Read the model definition and answer for the solid it produces. Units are mm, in the model's axes. A direction names the side the tool comes from. Coordinates: 2 decimals unless noted, no trailing zeros. Order: outer loops, then holes, each group sorted by start corner. A loop starts at its lowest first (then second) coordinate and runs counter-clockwise, first axis right, second up. Notation, with made-up numbers: (38.25, -22) -> (56.25, -22) arc R22 cw to (56.25, -5) -> close; hole circle Ø1 at (21.5, 23). An arc over 180 degrees is marked (long way). Answer in a Markdown table with one row per item.
from build123d import *
from build123d.topology import SkipClean

# Parameters (mm, degrees)
SKETCH_1_R               = 25
EXTRUDE_1_DEPTH          = 15
SKETCH_2_R               = 22.15
CUT_EXTRUDE_1_DEPTH      = 12.5
SKETCH_3_R               = 18.15
CUT_EXTRUDE_2_DEPTH      = 12.5
EXTRUDE_2_DEPTH          = 15
FILLET_1_R               = 8
CUT_EXTRUDE_START        = -15
SKETCH_5_R               = 1.5
CUT_EXTRUDE_3_DEPTH      = 15
SKETCH_6_R               = 3
CUT_EXTRUDE_4_DEPTH      = 2
PATTERN_CIRCULAR_1_COUNT = 4
CUT_EXTRUDE_5_DEPTH      = 10
FILLET_2_R               = 2


with BuildPart() as part:
    # 草图1 → 凸台-拉伸1 (new body)
    with BuildSketch(Plane(origin=(0, 0, 0), x_dir=(1, 0, 0), z_dir=(0, 1, 0))):
        with Locations(Location((0, 0, 0), (0, 0, 270))):
            Circle(SKETCH_1_R)
    extrude(amount=EXTRUDE_1_DEPTH)

    # 草图2 → 切除-拉伸1 (cut)
    with BuildSketch(Plane(origin=(0, 15, 0), x_dir=(1, 0, 0), z_dir=(0, 1, 0))):
        with Locations(Location((0, 0, 0), (0, 0, 270))):
            Circle(SKETCH_2_R)
    extrude(amount=-CUT_EXTRUDE_1_DEPTH, mode=Mode.SUBTRACT)

    # 草图3 → 切除-拉伸2 (cut)
    with BuildSketch(Plane(origin=(0, 2.5, 0), x_dir=(1, 0, 0), z_dir=(0, 1, 0))):
        with Locations(Location((0, 0, 0), (0, 0, 270))):
            Circle(SKETCH_3_R)
    extrude(amount=-CUT_EXTRUDE_2_DEPTH, mode=Mode.SUBTRACT)

    # 草图4 → 凸台-拉伸2 (add)
    with BuildSketch(Plane(origin=(0, 0, 0), x_dir=(1, 0, 0), z_dir=(0, 1, 0))):
        with BuildLine():
            Line((0, 25), (-25, 25))
            Line((-25, 25), (-25, 2.6e-08))
            ThreePointArc((-25, 2.6e-08), (-23.301207713, 9.058350794), (-18.435702489, 16.885641052))
            ThreePointArc((-18.435702489, 16.885641052), (-19.445436483, 19.445436483), (-16.885641052, 18.435702489))
            ThreePointArc((-16.885641052, 18.435702489), (-9.058350782, 23.301207718), (0, 25))
        make_face()
        with BuildLine():
            Line((25, 25), (0, 25))
            ThreePointArc((0, 25), (9.210354363, 23.241544108), (17.125028574, 18.213549801))
            ThreePointArc((17.125028574, 18.213549801), (19.682469279, 19.438809921), (18.425448396, 16.896829626))
            ThreePointArc((18.425448396, 16.896829626), (23.298457137, 9.065423048), (25, 0))
            Line((25, 0), (25, 25))
        make_face()
        with BuildLine():
            ThreePointArc((-18.213549801, -17.125028574), (-23.241544113, -9.210354351), (-25, 2.6e-08))
            Line((-25, 2.6e-08), (-25, -25))
            Line((-25, -25), (-5.8e-08, -25))
            ThreePointArc((-5.8e-08, -25), (-9.065423076, -23.298457126), (-16.896829626, -18.425448396))
            ThreePointArc((-16.896829626, -18.425448396), (-19.438809921, -19.682469279), (-18.213549801, -17.125028574))
        make_face()
        with BuildLine():
            Line((25, -25), (25, 0))
            ThreePointArc((25, 0), (23.22561674, -9.250444694), (18.154341838, -17.18778265))
            ThreePointArc((18.154341838, -17.18778265), (19.675883861, -19.675883861), (17.18778265, -18.154341838))
            ThreePointArc((17.18778265, -18.154341838), (9.250444666, -23.225616751), (-5.8e-08, -25))
            Line((-5.8e-08, -25), (25, -25))
        make_face()
    extrude(amount=EXTRUDE_2_DEPTH)

    # 圆角1
    fillet_1_edges = [part.edges().sort_by_distance(p)[0] for p in [
        (-25, 7.5, -25),
        (25, 7.5, -25),
        (-25, 7.5, 25),
        (25, 7.5, 25),
    ]]
    fillet(fillet_1_edges, radius=FILLET_1_R)

    # 草图5 → 切除-拉伸3 (cut)
    with BuildSketch(Plane(origin=(0, 15, 0), x_dir=(1, 0, 0), z_dir=(0, 1, 0)).offset(CUT_EXTRUDE_START)):
        with Locations(Location((-18.384776311, 18.384776311, 0), (0, 0, 270))):
            Circle(SKETCH_5_R)
        with Locations(Location((18.615223689, 18.384776311, 0), (0, 0, 270))):
            Circle(SKETCH_5_R)
        with Locations(Location((18.615223689, -18.615223689, 0), (0, 0, 270))):
            Circle(SKETCH_5_R)
        with Locations(Location((-18.384776311, -18.615223689, 0), (0, 0, 270))):
            Circle(SKETCH_5_R)
    extrude(amount=CUT_EXTRUDE_3_DEPTH, mode=Mode.SUBTRACT)

    # 草图6 → 切除-拉伸4 (cut)
    with BuildSketch(Plane(origin=(0, 15, 0), x_dir=(1, 0, 0), z_dir=(0, 1, 0))):
        with Locations(Location((-18.384776311, 18.384776311, 0), (0, 0, 270))):
            Circle(SKETCH_6_R)
    cut_extrude_4 = extrude(amount=-CUT_EXTRUDE_4_DEPTH, mode=Mode.SUBTRACT)

    # 阵列(圆周)1: 切除-拉伸4 ×4 about axis
    with SkipClean():  # the faces are left unmerged after this step: merging them gives an invalid solid
        pattern_circular_1_axis = Axis((0, 0, 0), (0, 1, 0))
        for i in range(1, PATTERN_CIRCULAR_1_COUNT):
            add(cut_extrude_4.rotate(pattern_circular_1_axis, i * 360 / PATTERN_CIRCULAR_1_COUNT), mode=Mode.SUBTRACT)

    # 草图7 → 切除-拉伸5 (cut)
    with SkipClean():  # the faces are left unmerged after this step: merging them gives an invalid solid
        with BuildSketch(Plane.XZ):
            Polygon((15.541599538, 17.817622342), (17.769154642, 15.554586419), (20.842778794, 16.352187766), (21.688847841, 19.412825036), (19.461292736, 21.67586096), (16.387668585, 20.878259612), align=None)
            Polygon((-15.32413904, 17.769154642), (-16.121740388, 20.842778794), (-19.182377658, 21.688847841), (-21.445413581, 19.461292736), (-20.647812234, 16.387668585), (-17.587174964, 15.541599538), align=None)
            Polygon((17.817622342, -15.311152159), (15.554586419, -17.538707264), (16.352187766, -20.612331415), (19.412825036, -21.458400462), (21.67586096, -19.230845358), (20.878259612, -16.157221206), align=None)
            Polygon((-15.311152159, -17.587174964), (-17.538707264, -15.32413904), (-20.612331415, -16.121740388), (-21.458400462, -19.182377658), (-19.230845358, -21.445413581), (-16.157221206, -20.647812234), align=None)
        extrude(amount=-CUT_EXTRUDE_5_DEPTH, mode=Mode.SUBTRACT)

    # 圆角2
    # the kernel refuses this fillet: 2 mm, written as the material it takes off along each edge
    with BuildSketch(Plane(origin=(0, 15, 0), x_dir=(0, 0, 1), z_dir=(-1, 0, 0))) as fillet_2_piece_1:
        with BuildLine():
            CenterArc((22.15 + FILLET_2_R, -FILLET_2_R), FILLET_2_R, 90, 90)
            Line((22.15, -FILLET_2_R), (22.15, 0))
            Line((22.15, 0), (22.15 + FILLET_2_R, 0))
        make_face()
    revolve(axis=Axis((0, 15, 0), (0, 1, 0)), mode=Mode.SUBTRACT)


solid = part.part
Q1. Consider line 1 (X direction, y = 10, z = 0); line 2 (X direction, y = 3.5, z = 18); line 3 (Z direction, x = -18, y = 4.5). Determine where each line is inside the solid, lowest interval first.
Outcome:
| item | result |
|---|---|
| line 1 | -25 to -22.15, 22.15 to 25 |
| line 2 | -24.94 to -21.07, -15.38 to -12.91, 12.91 to 15.59, 21.3 to 24.94 |
| line 3 | -24.94 to -21.13, -15.44 to -12.91, 12.91 to 15.66, 21.36 to 24.94 |
Q2. The part is cut by section D-D (y = 7.25). Give the number of separate pieces and of enclosed holes in the cut face, then the cut area to 3 significant figures.
Outcome:
| item | result |
|---|---|
| separate pieces | 1 |
| enclosed holes | 5 |
| area | 799 mm² |
Q3. The part is cut by section B-B (x = 0). Write down the section's boundary in (y, z), then the cut area to 3 significant figures.
Outcome:
| item | result |
|---|---|
| outline | (0, -25) -> (15, -25) -> (15, -24.15) arc R2 ccw to (13, -22.15) -> (2.5, -22.15) -> (2.5, -18.15) -> (0, -18.15) -> close; (0, 18.15) -> (2.5, 18.15) -> (2.5, 22.15) -> (13, 22.15) arc R2 ccw to (15, 24.15) -> (15, 25) -> (0, 25) -> close |
| area | 104 mm² |
Q4. The part is cut by section C-C (y = 12.25). Write down the section's boundary in (x, z).
Outcome:
| item | result |
|---|---|
| outline | (-25, -17) arc R8 ccw to (-17, -25) -> (17, -25) arc R8 ccw to (25, -17) -> (25, 17) arc R8 ccw to (17, 25) -> (-17, 25) arc R8 ccw to (-25, 17) -> close; hole circle Ø44.3 at (0, 0); hole circle Ø3 at (-18.38, -18.38); hole circle Ø3 at (-18.38, 18.62); hole circle Ø3 at (18.62, -18.38); hole circle Ø3 at (18.62, 18.62) |
Q5. Given pin 1 (1.8 mm diameter, centred on x = -20, z = -18, fed in from -Y); pin 2 (2.5 mm diameter, centred on x = -18.38, z = 18.62, fed in from -Y); pin 3 (3.5 mm diameter, centred on x = 18.62, z = 18.62, fed in from +Y), each flat-ended and moving along its own axis, determine where each tip first touches the part or whether it passes through.
Outcome:
| item | result |
|---|---|
| pin 1 | y = 10 |
| pin 2 | through |
| pin 3 | y = 13 |
Q6. For faces 3 (the face through (-20, 10, -18)), 4 (the face through (18, 13, 17)), determine the directions among +Z, -Z, +X, -X, +Y, -Y from which every point of the face is accessible in a straight line to the end or side of a thin tool.
Outcome:
| item | result |
|---|---|
| face 3 | -Y |
| face 4 | +Y |
Q7. For a pull along Z with two mould halves and no side action, classify faces 1 (the face through (-22.594, 7.605, -22.719)), 2 (the face through (-20.36, 4.93, -20.3)) as pulls with the +Z half, pulls with the -Z half, needs draft (parallel to the pull), parting line crosses it, or undercut.
Outcome:
| item | result |
|---|---|
| face 1 | pulls with the -Z half |
| face 2 | undercut |
Q8. The part is cut by section A-A (z = 0). Write down the section's boundary in (x, y), then the cut area to 3 significant figures.
Outcome:
| item | result |
|---|---|
| outline | (-25, 0) -> (-18.15, 0) -> (-18.15, 2.5) -> (-22.15, 2.5) -> (-22.15, 13) arc R2 ccw to (-24.15, 15) -> (-25, 15) -> close; (18.15, 0) -> (25, 0) -> (25, 15) -> (24.15, 15) arc R2 ccw to (22.15, 13) -> (22.15, 2.5) -> (18.15, 2.5) -> close |
| area | 104 mm² |
